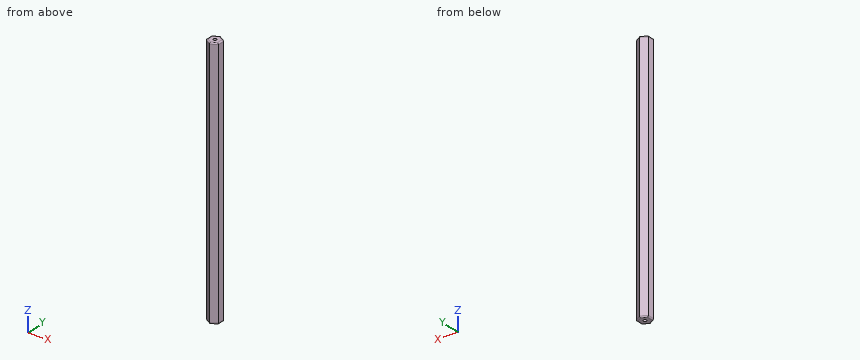
from build123d import *

# Parameters (mm, degrees)
RESSALTO_EXTRUS_O1_DEPTH = 105
FILETE1_R                = 0.5
ESBO_O2_R                = 0.701481341
CORTE_EXTRUS_O1_DEPTH    = 106


with BuildPart() as part:
    # Esboço1 → Ressalto-extrusão1 (new body)
    with BuildSketch(Plane.XY.offset(135)):
        Polygon((-55.002122675, 2.886751346), (-57.502122675, 1.443375673), (-57.502122675, -1.443375673), (-55.002122675, -2.886751346), (-52.502122675, -1.443375673), (-52.502122675, 1.443375673), align=None)
    extrude(amount=-RESSALTO_EXTRUS_O1_DEPTH)

    # Filete1
    filete1_edges = [part.edges().sort_by_distance(p)[0] for p in [
        (-57.502122675, 0, 30),
        (-56.252122675, -2.165063509, 30),
        (-53.752122675, -2.165063509, 30),
        (-52.502122675, 0, 30),
        (-53.752122675, 2.165063509, 30),
        (-52.502122675, 0, 135),
        (-53.752122675, -2.165063509, 135),
        (-56.252122675, -2.165063509, 135),
        (-57.502122675, 0, 135),
        (-56.252122675, 2.165063509, 135),
        (-53.752122675, 2.165063509, 135),
        (-56.252122675, 2.165063509, 30),
    ]]
    fillet(filete1_edges, radius=FILETE1_R)

    # Esboço2 → Corte-extrusão1 (cut, through all)
    with BuildSketch(Plane.XY.offset(135)):
        with Locations((-55.002122675, 0)):
            Circle(ESBO_O2_R)
    extrude(amount=-CORTE_EXTRUS_O1_DEPTH, mode=Mode.SUBTRACT)


solid = part.part
The listing builds one solid part. Answer for the finished solid, in the listing's coordinates (mm). Give positions to 0.01 mm unless a question says otherwise; leave off trailing zeros. Order: outer loops, then holes, each group sorted by start corner. A loop starts at its lowest first (then second) coordinate and runs counter-clockwise, first axis right, second up. Notation, with made-up numbers: (24.5, 83.5) -> (64.5, 83.5) arc R22 cw to (64.5, 119.5) -> close; hole circle Ø6 at (70, -33.75). An arc over 180 degrees is marked (long way). Put each result on its own line as item: value.
Item 1: A cutting plane is placed at A-A on z = 95. Give the vertices of the cut face in (x, y).
Established:
outline: (-57.5, -1.44) -> (-55, -2.89) -> (-52.5, -1.44) -> (-52.5, 1.44) -> (-55, 2.89) -> (-57.5, 1.44) -> close; hole circle Ø1.4 at (-55, 0)
Item 2: Given P1, Ø2, axis at x = -55.5, z = 46, coming from the -Y side, flat-ended and moving along its own axis, determine where the tip first touches the part or whether it passes through.
Established:
P1: stops at y = -2.89
Item 3: Straight lines are drawn through the part: line 1 (Z direction, x = -53.45, y = 1.5); line 2 (Y direction, x = -55.45, z = 47.5); line 3 (X direction, y = -0.55, z = 67.5). For each, find the intervals that lie inside material, in ascending order.
Established:
line 1: z = 30.01 to 134.99
line 2: y = -2.63 to -0.54, 0.54 to 2.63
line 3: x = -57.5 to -55.44, -54.57 to -52.5
